Source: CAD feature listing. Evaluate the final solid. Frame: model axes, mm. Face numbers are marked on the shaded views. A direction names the side the tool comes from. Give positions to 0.01 mm unless a question says otherwise; leave off trailing zeros. Loops run counter-clockwise (first coordinate to the right, second up) from the corner with the lowest first, then second, coordinate; pieces in that order, holes last. Notation, with made-up numbers: M 32.25,73 L 49.25,73 A28 cw 49.25,111 Z; hole C 79.25,63.25 d2. An arc over 180 degrees is marked long. Answer in a Markdown table with one row per item.
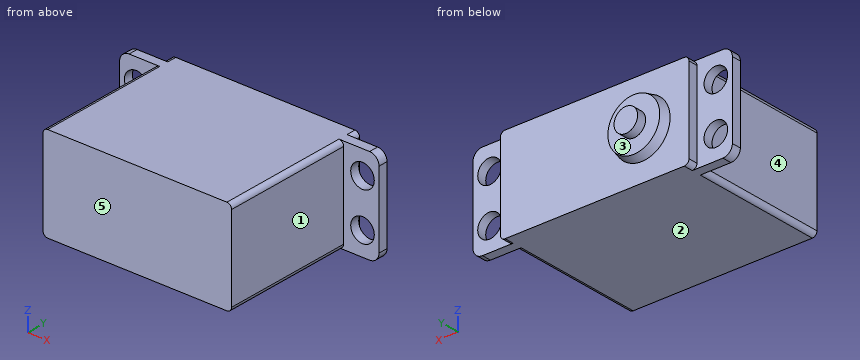
```python
from build123d import *

# Parameters (mm, degrees)
SKETCH1_W           = 55
SKETCH1_H           = 20
SKETCH1_R           = 2.5
BOSS_EXTRUDE1_DEPTH = 2
FILLET1_R           = 2
SKETCH2_W           = 40
SKETCH2_H           = 20
BOSS_EXTRUDE2_DEPTH = 28
SKETCH3_W           = 40
SKETCH3_H           = 20
BOSS_EXTRUDE3_DEPTH = 2
FILLET2_R           = 1


with BuildPart() as part:
    # Sketch1 → Boss-Extrude1 (new body)
    with BuildSketch(Plane(origin=(0, 0, 0), x_dir=(1, 0, 0), z_dir=(0, 1, 0))):
        with Locations((27.5, 10)):
            Rectangle(SKETCH1_W, SKETCH1_H)
        with Locations(Location((3.5, 15, 0), (0, 0, 270))):
            Circle(SKETCH1_R, mode=Mode.SUBTRACT)
        with Locations(Location((3.5, 5, 0), (0, 0, 270))):
            Circle(SKETCH1_R, mode=Mode.SUBTRACT)
        with Locations(Location((51.5, 15, 0), (0, 0, 270))):
            Circle(SKETCH1_R, mode=Mode.SUBTRACT)
        with Locations(Location((51.5, 5, 0), (0, 0, 270))):
            Circle(SKETCH1_R, mode=Mode.SUBTRACT)
    extrude(amount=BOSS_EXTRUDE1_DEPTH)

    # Fillet1
    fillet1_edges = [part.edges().sort_by_distance(p)[0] for p in [
        (0, 1, -20),
        (55, 1, -20),
        (55, 1, 0),
        (0, 1, 0),
    ]]
    fillet(fillet1_edges, radius=FILLET1_R)

    # Sketch2 → Boss-Extrude2 (add)
    with BuildSketch(Plane.XZ):
        with Locations((27.5, -10)):
            Rectangle(SKETCH2_W, SKETCH2_H)
    extrude(amount=BOSS_EXTRUDE2_DEPTH)

    # Sketch3 → Boss-Extrude3 (add)
    with BuildSketch(Plane(origin=(0, 2, 0), x_dir=(1, 0, 0), z_dir=(0, 1, 0))):
        with Locations((27.5, 10)):
            Rectangle(SKETCH3_W, SKETCH3_H)
    extrude(amount=BOSS_EXTRUDE3_DEPTH)

    # Fillet2
    fillet2_edges = [part.edges().sort_by_distance(p)[0] for p in [
        (7.5, -14, 0),
        (7.5, -14, -20),
        (47.5, -14, -20),
        (47.5, -14, 0),
        (7.5, 3, -20),
        (7.5, 3, 0),
        (47.5, 3, 0),
        (47.5, 3, -20),
    ]]
    fillet(fillet2_edges, radius=FILLET2_R)

    # Sketch4 → Revolve1 (revolve)
    with BuildSketch(Plane.XY.offset(-10), mode=Mode.PRIVATE) as revolve1_sk:
        Polygon((17.5, 4), (11.5, 4), (12, 6), (15, 6), (15, 8), (17.5, 8), align=None)
    revolve(revolve1_sk.sketch.rotate(Axis((17.5, 8, -10), (0, -1, 0)), 270), axis=Axis((17.5, 8, -10), (0, -1, 0)))


solid = part.part
```
Q1. Section query C-C (x = 17.5). Output: boundary loops of the cut face in (y, z).
Values follow:
| item | result |
|---|---|
| outline | M -28,-20 L 4,-20 L 4,-16 L 6,-15.5 L 6,-12.5 L 8,-12.5 L 8,-7.5 L 6,-7.5 L 6,-4.5 L 4,-4 L 4,0 L -28,0 Z |
Q2. Contact query for flat-ended pins moving along their axis: pin 1 Ø6 at (x, z) = (31, -11.5) entering from +Y; pin 2 Ø1 at (y, z) = (-19.5, -17) entering from -X; pin 3 Ø4 at (x, z) = (3.5, -9) entering from +Y. Output: stop coordinate, or through.
Values follow:
| item | result |
|---|---|
| pin 1 | y = 4 |
| pin 2 | x = 7.5 |
| pin 3 | y = 2 |
Q3. Section query A-A (x = 51.5). Output: boundary loops of the cut face in (y, z), plus the area to 3 significant figures.
Values follow:
| item | result |
|---|---|
| outline | M 0,-20 L 2,-20 L 2,-17.5 L 0,-17.5 Z; M 0,-12.5 L 2,-12.5 L 2,-7.5 L 0,-7.5 Z; M 0,-2.5 L 2,-2.5 L 2,0 L 0,0 Z |
| area | 20.0 mm^2 |
Q4. Section query D-D (y = -3.5). Output: boundary loops of the cut face in (x, z), plus the area to 3 significant figures.
Values follow:
| item | result |
|---|---|
| outline | M 7.5,-19 A1 ccw 8.5,-20 L 46.5,-20 A1 ccw 47.5,-19 L 47.5,-1 A1 ccw 46.5,0 L 8.5,0 A1 ccw 7.5,-1 Z |
| area | 799 mm^2 |
Q5. Section query B-B (z = -10). Output: boundary loops of the cut face in (x, y), plus the area to 3 significant figures.
Values follow:
| item | result |
|---|---|
| outline | M 0,0 L 7.5,0 L 7.5,-28 L 47.5,-28 L 47.5,0 L 55,0 L 55,2 L 47.5,2 L 47.5,4 L 23.5,4 L 23,6 L 20,6 L 20,8 L 15,8 L 15,6 L 12,6 L 11.5,4 L 7.5,4 L 7.5,2 L 0,2 Z |
| area | 1,340 mm^2 |
Q6. Reachability of the marked faces 1, 2, 3, 4 and 5 from +Z, -Z, +X, -X, +Y, -Y: full face, straight path, thin tool, end or side. Return the list, or none.
Values follow:
| item | result |
|---|---|
| face 1 | +Z, -Z, +X, -Y |
| face 2 | -Z, +X, -X, +Y, -Y |
| face 3 | +Y |
| face 4 | +Z, -Z, -X, -Y |
| face 5 | +Z, -Z, +X, -X, -Y |
Q7. Ray query, probe 1 along X at (y, z) = (0.65, -5); probe 2 along Z at (x, y) = (3, 1); probe 3 along X at (y, z) = (1, -14). Return the intervals inside material, ascending. Write a range as from..to.
Values follow:
| item | result |
|---|---|
| probe 1 | 0..1, 6..49, 54..55 |
| probe 2 | -20..-17.45, -12.55..-7.45, -2.55..0 |
| probe 3 | 0..1.21, 5.79..49.21, 53.79..55 |
